from build123d import *

# Parameters (mm, degrees)
F1_DEPTH = 41.91
F2_R     = 4.6355
F3_DEPTH = 2.032
F4_DEPTH = 3.048
F5_DEPTH = 1.778


with BuildPart() as f1:
    # F0 (on Right) → F1 (new body)
    with BuildSketch(Plane.YZ):
        Polygon((50.8, 0), (0, 0), (-14.3346570664, -81.2958800112), (0, -81.2958800112), align=None)
    extrude(amount=-F1_DEPTH)

    # F2 (on face) → F3 (join)
    with BuildSketch(Plane(origin=(0, 0, 0), x_dir=(1, 0, 0), z_dir=(0, -0.984807753, 0.1736481777))):
        with Locations((-20.955, -40.64)):
            Circle(F2_R)
    extrude(amount=F3_DEPTH)

    # F2 (on face) → F4 (join)
    with BuildSketch(Plane(origin=(0, 0, 0), x_dir=(1, 0, 0), z_dir=(0, -0.984807753, 0.1736481777))):
        with BuildLine():
            ThreePointArc((-8.2651640673, -34.798), (-6.985, -40.64), (-8.2651640673, -46.482))
            Line((-8.2651640673, -46.482), (-4.4986959724, -46.482))
            ThreePointArc((-4.4986959724, -46.482), (-3.4925, -40.64), (-4.4986959724, -34.798))
            Line((-4.4986959724, -34.798), (-8.2651640673, -34.798))
        make_face()
        with BuildLine():
            ThreePointArc((-4.4986959724, -34.798), (-3.4925, -40.64), (-4.4986959724, -46.482))
            Line((-4.4986959724, -46.482), (-3.2235985607, -46.482))
            ThreePointArc((-3.2235985607, -46.482), (-2.286, -40.64), (-3.2235985607, -34.798))
            Line((-3.2235985607, -34.798), (-4.4986959724, -34.798))
        make_face()
    extrude(amount=F4_DEPTH)

    # F2 (on face) → F5 (cut)
    with BuildSketch(Plane(origin=(0, 0, 0), x_dir=(1, 0, 0), z_dir=(0, -0.984807753, 0.1736481777))):
        with BuildLine():
            ThreePointArc((-4.4986959724, -34.798), (-3.4925, -40.64), (-4.4986959724, -46.482))
            Line((-4.4986959724, -46.482), (-3.2235985607, -46.482))
            ThreePointArc((-3.2235985607, -46.482), (-2.286, -40.64), (-3.2235985607, -34.798))
            Line((-3.2235985607, -34.798), (-4.4986959724, -34.798))
        make_face()
    extrude(amount=F5_DEPTH, mode=Mode.SUBTRACT)

    # F7: F1 across plane


with BuildPart() as f1_1:
    add(f1.part)
    add(f1.part.mirror(Plane(origin=(-20.955, 12.1551143112, -33.0624182644), x_dir=(0, 1, 0), z_dir=(1, 0, 0))))


solid = f1_1.part
Build history of the part. All positions in model axes, mm. A direction names the side the tool comes from. Coordinates: 2 decimals unless noted, no trailing zeros. Order: outer loops, then holes, each group sorted by start corner. A loop starts at its lowest first (then second) coordinate and runs counter-clockwise, first axis right, second up. Notation, with made-up numbers: (-16, -8.75) - (-2, -8.75) arc R9 cw to (-2, 4.25) - close; hole circle Ø5 at (11, 67). An arc over 180 degrees is marked (long way). Write each question's results on one line, items separated by ' | '. Start each with the question number.
Item 1: Band-saw the part on C-C on z = -47. Write the cut outline in (x, y), and give its area (3 significant figures).
Item 2: Wall check: probe 1 along X at (y, z) = (-8, -39); probe 2 along Z at (x, y) = (-3.5, 12); probe 3 along Y at (x, z) = (-12, -59). Give the ranges that are in metal, low to high. Write a range as [from, to].
Item 3: Mould opens along X. For faces 1 (the face through (0, 11, -31)), 2 (the face through (-21.02, -9.047, -39.606)), 3 (the face through (-21, -7, -81.296)), 4 (the face through (-41.91, 11, -31)) say: released by +X, released by -X, zero draft, split by the parting line, or undercut.
Item 4: Band-saw the part on A-A on x = -36.5. Write the cut outline in (y, z).
Item 5: Band-saw the part on B-B on y = 18. Write the cut outline in (x, z), and give its area (3 significant figures).
Item 6: Tool access for faces 5 (the face through (-38.748, -8.794, -39.633)), 6 (the face through (-36.13, -9.551, -45.515)), 7 (the face through (-5.71, -7.52, -34.01)), 8 (the face through (-6.985, -8.522, -39.679)): list every direction of +Z, -Z, +X, -X, +Y, -Y with a clear straight run to the whole face (end or side of a thin tool).
Item 7: Flat gauge pins, fed straight in: pin 1 (5 mm diameter, centred on x = -10.5, z = -62, fed in from +Y); pin 2 (12 mm diameter, centred on x = -25.5, z = -42.5, fed in from -Y); pin 3 (2 mm diameter, centred on x = -9.5, y = 42, fed in from -Z). Where does each tip first touch, or does it go through?
Numbers:
1) outline: (-41.91, -8.29) - (0, -8.29) - (0, 21.43) - (-41.91, 21.43) - close | area: 1,250 mm^2
2) probe 1: [-38.4, -34.9], [-25.51, -16.4], [-7.01, -3.51] | probe 2: [-62.09, 0] | probe 3: [-10.4, 13.93]
3) face 1: released by +X | face 2: undercut | face 3: zero draft | face 4: released by -X
4) outline: (-14.33, -81.3) - (0, -81.3) - (50.8, 0) - (0, 0) - (-6.04, -34.27) - (-9.04, -33.74) - (-11.07, -45.25) - (-8.07, -45.78) - close
5) outline: (-41.91, -52.49) - (0, -52.49) - (0, 0) - (-41.91, 0) - close | area: 2,200 mm^2
6) face 5: -X | face 6: +X, -X, -Y | face 7: +Z, +X, -X | face 8: none
7) pin 1: y = 13.62 | pin 2: y = -9.86 | pin 3: z = -15.68
